Design review of the part built by this model. Coordinates are the model's own, in mm. A direction names the side the tool comes from. Round coordinates to 2 decimals unless told otherwise and drop trailing zeros. Order: outer loops, then holes, each group sorted by start corner. A loop starts at its lowest first (then second) coordinate and runs counter-clockwise, first axis right, second up. Notation, with made-up numbers: M -26,87 L 10,87 A13 ccw 10,98 Z; hole C -34,31 d7. An arc over 180 degrees is marked long. Use a Markdown table: item, result. Add a question column.
(1) Take a section at A-A (y = 25). Write out the cut boundary in (x, z), then the cut area to 3 significant figures.
(2) Machinability: for faces 1 (the face through (-8.886, 38, 1)), 2 (the face through (39.182, -18, 1)), which of the approach directions +Z, -Z, +X, -X, +Y, -Y give a long, thin tool a straight path to every point of the face, cutting with its end or side? Answer none if there is none.
(3) The part is to be moulded in two halves that separate along X. For faces 3 (the face through (13.233, -23.687, 1.479)), 4 (the face through (37.348, -11.303, 1.479)), 5 (the face through (-37.288, -11.335, 1.479)), say which applies: released by +X, released by -X, zero draft, split by the parting line, or undercut.
(4) To check wall thickness, follow probe 1 along Y at (x, z) = (21, 0.2); probe 2 along X at (y, z) = (-21, 0.75); probe 3 along X at (y, z) = (-22.5, 1.25). State the ranges of each line that lie inside material, in increasing order. Write a range as from..to.
(5) Take a section at B-B (z = 1.15). Write out the cut boundary in (x, y).
(6) For pin 1 (1 mm diameter, centred on x = -25, z = 2.5, fed in from +Y); pin 2 (1.5 mm diameter, centred on y = 37, z = 1.5, fed in from -X); pin 3 (1 mm diameter, centred on y = 20, z = 1, fed in from -X), all flat-tipped, find the tip position at first contact; note any pin that passes through.
(7) Take a section at D-D (y = -17). Write out the cut boundary in (x, z), then the cut area to 3 significant figures.
(8) Take a section at C-C (x = 29). Write out the cut boundary in (y, z).
```python
from build123d import *

# Parameters (mm, degrees)
F0_R     = 11
F1_DEPTH = 3


with BuildPart() as f1:
    # F0 (on Top) → F1 (new body)
    with BuildSketch(Plane.XY):
        with BuildLine():
            ThreePointArc((-26.5772530672, -25.6045196536), (-13.359413403, -23.7807642853), (-7.6729374941, -11.710082417))
            ThreePointArc((-7.6729374941, -11.710082417), (-4.0036761959, -13.4153112867), (0, -14))
            ThreePointArc((0, -14), (4.0036761959, -13.4153112867), (7.6729374941, -11.710082417))
            ThreePointArc((7.6729374941, -11.710082417), (13.3895340738, -23.80284079), (26.6470947033, -25.5780499838))
            Line((26.6470947033, -25.5780499838), (30.3253398397, -27.7016858035))
            Line((30.3253398397, -27.7016858035), (39.1819556656, -22.5883162723))
            Line((39.1819556656, -22.5883162723), (39.1819556656, -12.3615772099))
            Line((39.1819556656, -12.3615772099), (35.4627910053, -10.2143164922))
            ThreePointArc((35.4627910053, -10.2143164922), (27.274452694, 0.320790756), (13.9776976005, -0.789917583))
            ThreePointArc((13.9776976005, -0.789917583), (13.6198384719, 3.2403703492), (12.124355653, 7))
            ThreePointArc((12.124355653, 7), (9.616162276, 10.1749409375), (6.3047601065, 12.5))
            ThreePointArc((6.3047601065, 12.5), (13.9190977695, 23.4970970478), (8.8276937136, 35.866085942))
            Line((8.8276937136, 35.866085942), (8.8276937136, 40.1133575813))
            Line((8.8276937136, 40.1133575813), (-0.0289221123, 45.2267271125))
            Line((-0.0289221123, 45.2267271125), (-8.8855379381, 40.1133575813))
            Line((-8.8855379381, 40.1133575813), (-8.8855379381, 35.8188361458))
            ThreePointArc((-8.8855379381, 35.8188361458), (-13.915039291, 23.4599735294), (-6.3047601065, 12.5))
            ThreePointArc((-6.3047601065, 12.5), (-9.616162276, 10.1749409375), (-12.124355653, 7))
            ThreePointArc((-12.124355653, 7), (-13.6198384719, 3.2403703492), (-13.9776976005, -0.789917583))
            ThreePointArc((-13.9776976005, -0.789917583), (-27.3086318433, 0.3057437422), (-35.4747884169, -10.2880359582))
            Line((-35.4747884169, -10.2880359582), (-39.1530335533, -12.4116717778))
            Line((-39.1530335533, -12.4116717778), (-39.1530335533, -22.6384108402))
            Line((-39.1530335533, -22.6384108402), (-30.2964177275, -27.7517803714))
            Line((-30.2964177275, -27.7517803714), (-26.5772530672, -25.6045196536))
        make_face()
        with Locations((-21.6506350946, -12.5)):
            Circle(F0_R, mode=Mode.SUBTRACT)
        with BuildLine():
            ThreePointArc((0, -11), (-9.5262794416, -5.5), (-9.5262794416, 5.5))
            ThreePointArc((-9.5262794416, 5.5), (0, 11), (9.5262794416, 5.5))
            ThreePointArc((9.5262794416, 5.5), (9.5262794416, -5.5), (0, -11))
        make_face(mode=Mode.SUBTRACT)
        with Locations((21.6506350946, -12.5)):
            Circle(F0_R, mode=Mode.SUBTRACT)
        with Locations((0, 25)):
            Circle(F0_R, mode=Mode.SUBTRACT)
    extrude(amount=F1_DEPTH)


solid = f1.part
```
Verdict:
| question | item | result |
|---|---|---|
| 1 | outline | M -14,0 L -11,0 L -11,3 L -14,3 Z; M 11,0 L 14,0 L 14,3 L 11,3 Z |
| 1 | area | 18.0 mm^2 |
| 2 | face 1 | +Z, -Z, -X, +Y |
| 2 | face 2 | +Z, -Z, +X, +Y, -Y |
| 3 | face 3 | undercut |
| 3 | face 4 | released by +X |
| 3 | face 5 | released by -X |
| 4 | probe 1 | y = -26.48..-23.48, -1.52..1.48 |
| 4 | probe 2 | x = -39.15..-28.63, -14.67..-10.53, 10.53..14.67, 28.63..39.18 |
| 4 | probe 3 | x = -39.15..-26.23, -17.07..-11.85, 11.85..17.07, 26.23..39.18 |
| 5 | outline | M -39.15,-22.64 L -30.3,-27.75 L -26.58,-25.6 A14 ccw -7.67,-11.71 A14 ccw 7.67,-11.71 A14 ccw 26.65,-25.58 L 30.33,-27.7 L 39.18,-22.59 L 39.18,-12.36 L 35.46,-10.21 A14 ccw 13.98,-0.79 A14 ccw 6.3,12.5 A14 ccw 8.83,35.87 L 8.83,40.11 L -0.03,45.23 L -8.89,40.11 L -8.89,35.82 A14 ccw -6.3,12.5 A14 ccw -13.98,-0.79 A14 ccw -35.47,-10.29 L -39.15,-12.41 Z; hole C -21.65,-12.5 d22; hole C 0,0 d22; hole C 0,25 d22; hole C 21.65,-12.5 d22 |
| 6 | pin 1 | stops at y = 1.21 |
| 6 | pin 2 | stops at x = -8.89 |
| 6 | pin 3 | stops at x = -13.26 |
| 7 | outline | M -39.15,0 L -31.69,0 L -31.69,3 L -39.15,3 Z; M -11.61,0 L -8.39,0 L -8.39,3 L -11.61,3 Z; M 8.39,0 L 11.61,0 L 11.61,3 L 8.39,3 Z; M 31.69,0 L 39.18,0 L 39.18,3 L 31.69,3 Z |
| 7 | area | 64.2 mm^2 |
| 8 | outline | M -26.94,0 L -20.68,0 L -20.68,3 L -26.94,3 Z; M -4.32,0 L -0.58,0 L -0.58,3 L -4.32,3 Z |
